Verification items for the finished model (mm, model axes). A direction names the side the tool comes from. Give positions to 0.01 mm unless a question says otherwise; leave off trailing zeros. Order: outer loops, then holes, each group sorted by start corner. A loop starts at its lowest first (then second) coordinate and runs counter-clockwise, first axis right, second up. Notation, with made-up numbers: (28.25, 8.5) -> (50.25, 8.5) arc R29 cw to (50.25, 29.5) -> close; hole circle Ø6 at (52, 60.5). An arc over 180 degrees is marked (long way). One line per question, with ' | ' between items. Start each with the question number.
Q1. Section check C-C on x = -35.5. Record the cut outline in (y, z), plus the area to 3 significant figures.
Q2. Mould release check, pull along X, two halves, no side actions. Record for faces 4 (the flat face through (1, 8, 57)), 5 (the flat face through (-73, 11, 20)): released by +X, released by -X, zero draft, split by the parting line, or undercut.
Q3. Section check D-D on y = 69. Record the cut outline in (x, z).
Q4. Section check B-B on y = 8. Record the cut outline in (x, z).
Q5. Section check A-A on x = 73. Record the cut outline in (y, z).
Q6. Material ranges on probe 1 along Z at (x, y) = (0, 72); probe 2 along Y at (x, z) = (-43, -22); probe 3 along Y at (x, z) = (84, -41), recorded low to high. Write a range as [from, to].
Q7. Access from +Z, -Z, +X, -X, +Y, -Y to the whole of each face (thin tool, end or side, straight path). Record for faces 1 (the cylindrical face through (4.036, 22.409, 30.736)), 2 (the cylindrical face through (-84, 11, -28)), 3 (the flat face through (50, 3, 1)).
Q8. Go/stop test with flat-tipped pins: pin 1 (19 mm diameter, centred on x = -68.5, z = -23, fed in from +Y); pin 2 (2.5 mm diameter, centred on x = -23.5, z = -2, fed in from +Y); pin 3 (3 mm diameter, centred on y = 63.5, z = -23, fed in from +X). Record where each tip stops, or that it passes through.
from build123d import *

# Parameters (mm, degrees)
BOSS_EXTRUDE1_DEPTH = 57
SKETCH2_W           = 85.5
SKETCH2_H           = 94
CUT_EXTRUDE1_DEPTH  = 3
SKETCH5_R           = 19
BOSS_EXTRUDE4_DEPTH = 3
CUT_EXTRUDE3_DEPTH  = 20
SKETCH7_R           = 47.5
SKETCH7_R_2         = 31
BOSS_EXTRUDE5_DEPTH = 61
SKETCH12_W          = 3
SKETCH12_H          = 37
SKETCH17_R          = 1.5
CUT_EXTRUDE4_DEPTH  = 10


with BuildPart() as part:
    # Sketch1 → Boss-Extrude1 (new body, symmetric)
    with BuildSketch(Plane.XY):
        Polygon((102, 0), (-102, 0), (-98.482758621, 16), (98.482758621, 16), align=None)
    extrude(amount=BOSS_EXTRUDE1_DEPTH, both=True)

    # Sketch2 → Cut-Extrude1 (cut)
    with BuildSketch(Plane.XZ):
        with Locations((-49.25, 0)):
            Rectangle(SKETCH2_W, SKETCH2_H)
    cut_extrude1 = extrude(amount=-CUT_EXTRUDE1_DEPTH, mode=Mode.SUBTRACT)

    # Mirror1: Cut-Extrude1 across plane
    add(cut_extrude1.mirror(Plane(origin=(0, 0, 0), x_dir=(0, 0, 1), z_dir=(1, 0, 0))), mode=Mode.SUBTRACT)

    # Sketch5 → Boss-Extrude4 (add)
    with BuildSketch(Plane(origin=(0, 16, 0), x_dir=(1, 0, 0), z_dir=(0, 1, 0))):
        with Locations((-73, 28)):
            Circle(SKETCH5_R)
        with Locations((-73, -28)):
            Circle(SKETCH5_R)
    boss_extrude4 = extrude(amount=BOSS_EXTRUDE4_DEPTH)

    # Sketch6 → Cut-Extrude3 (cut, through all)
    with BuildSketch(Plane(origin=(0, 19, 0), x_dir=(1, 0, 0), z_dir=(0, 1, 0))):
        with BuildLine():
            Line((-76, 36), (-70, 36))
            ThreePointArc((-70, 36), (-62, 28), (-70, 20))
            Line((-70, 20), (-76, 20))
            ThreePointArc((-76, 20), (-84, 28), (-76, 36))
        make_face()
        with BuildLine():
            Line((-76, -20), (-70, -20))
            ThreePointArc((-70, -20), (-62, -28), (-70, -36))
            Line((-70, -36), (-76, -36))
            ThreePointArc((-76, -36), (-84, -28), (-76, -20))
        make_face()
    cut_extrude3 = extrude(amount=-CUT_EXTRUDE3_DEPTH, mode=Mode.SUBTRACT)

    # Mirror2: Boss-Extrude4, Cut-Extrude3 across plane
    add(boss_extrude4.mirror(Plane(origin=(0, 0, 0), x_dir=(0, 0, 1), z_dir=(1, 0, 0))))
    add(cut_extrude3.mirror(Plane(origin=(0, 0, 0), x_dir=(0, 0, 1), z_dir=(1, 0, 0))), mode=Mode.SUBTRACT)

    # Sketch7 → Boss-Extrude5 (add)
    with BuildSketch(Plane(origin=(0, 16, 0), x_dir=(1, 0, 0), z_dir=(0, 1, 0))):
        Circle(SKETCH7_R)
        with Locations(Location((0, 0, 0), (0, 0, 180))):  # turned: the seam where the file's is
            Circle(SKETCH7_R_2, mode=Mode.SUBTRACT)
    extrude(amount=BOSS_EXTRUDE5_DEPTH)

    # Sketch12 → Cut-Revolve6 (revolve, cut)
    with BuildSketch(Plane.XY, mode=Mode.PRIVATE) as cut_revolve6_sk:
        with Locations((-31, 47.5)):
            Rectangle(SKETCH12_W, SKETCH12_H)
    revolve(cut_revolve6_sk.sketch.rotate(Axis((0, 0, 0), (0.010431918, 0.999945586, 0)), 180), axis=Axis((0, 0, 0), (0.010431918, 0.999945586, 0)), mode=Mode.SUBTRACT)  # turned: the seam where the file's is

    # Sketch17 → Cut-Extrude4 (cut)
    with BuildSketch(Plane(origin=(0, 16, 0), x_dir=(1, 0, 0), z_dir=(0, 1, 0))):
        with Locations(Location((-23.5, 2.202781608, 0), (0, 0, 180))):  # turned: the seam where the file's is
            Circle(SKETCH17_R)
    extrude(amount=-CUT_EXTRUDE4_DEPTH, mode=Mode.SUBTRACT)


solid = part.part
Filled in:
1) outline: (0, -57) -> (16, -57) -> (16, -31.56) -> (77, -31.56) -> (77, 31.56) -> (16, 31.56) -> (16, 57) -> (0, 57) -> (0, 47) -> (3, 47) -> (3, -47) -> (0, -47) -> close | area: 5,390 mm²
2) face 4: zero draft | face 5: undercut
3) outline: circle Ø95 at (0, 0); hole circle Ø62 at (0, 0)
4) outline: (-100.24, -57) -> (100.24, -57) -> (100.24, 57) -> (-100.24, 57) -> close; hole (-76, -36) -> (-70, -36) arc R8 ccw to (-70, -20) -> (-76, -20) arc R8 ccw to start; hole (-76, 20) -> (-70, 20) arc R8 ccw to (-70, 36) -> (-76, 36) arc R8 ccw to start; hole circle Ø3 at (-23.5, -2.2); hole (70, -36) -> (76, -36) arc R8 ccw to (76, -20) -> (70, -20) arc R8 ccw to start; hole (70, 20) -> (76, 20) arc R8 ccw to (76, 36) -> (70, 36) arc R8 ccw to start
5) outline: (0, -57) -> (16, -57) -> (16, -47) -> (19, -47) -> (19, -36) -> (3, -36) -> (3, -47) -> (0, -47) -> close; (0, 47) -> (3, 47) -> (3, 36) -> (19, 36) -> (19, 47) -> (16, 47) -> (16, 57) -> (0, 57) -> close; (3, -20) -> (19, -20) -> (19, -9) -> (16, -9) -> (16, 9) -> (19, 9) -> (19, 20) -> (3, 20) -> close
6) probe 1: [-47.5, -31], [31, 47.5] | probe 2: [3, 16] | probe 3: [3, 19]
7) face 1: +Y | face 2: +Y, -Y | face 3: -Y
8) pin 1: y = 19 | pin 2: y = 6 | pin 3: x = 42.36
